Part print with two shaded views. Sizes in mm from the minimum x, y, z corner. A direction names the side the tool comes from. Coordinates: 2 decimals unless noted, no trailing zeros. Loops run counter-clockwise (first coordinate to the right, second up) from the corner with the lowest first, then second, coordinate; pieces in that order, holes last. Notation, with made-up numbers: (-3, 58) -> (11, 58) arc R26 cw to (11, 86) -> close; hole circle Ø3 at (-35, 83.25). An arc over 180 degrees is marked (long way). Write each question's results on one line, items separated by ' | '.
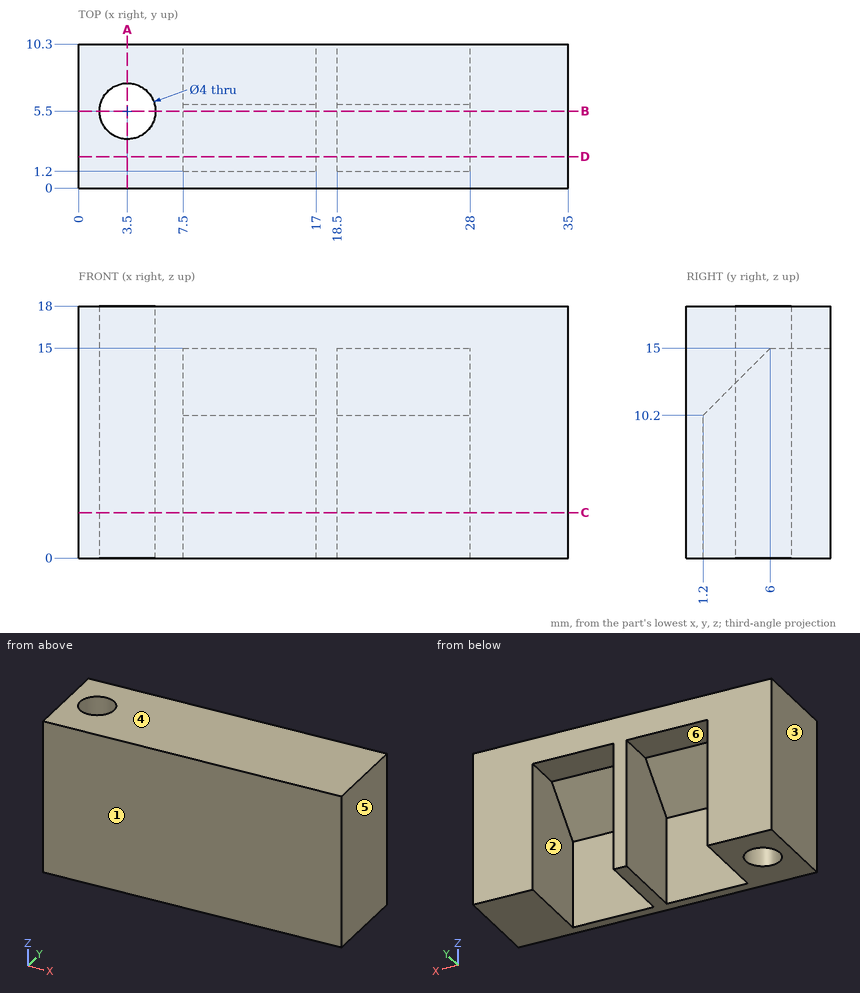
Q1. Drop flat-ended pins along their axis: pin 1 (5 mm diameter, centred on x = 12, z = 6, fed in from +Y); pin 2 (7.5 mm diameter, centred on x = 25, z = 4, fed in from +Y); pin 3 (2 mm diameter, centred on x = 13, y = 9, fed in from -Z); pin 4 (3 mm diameter, centred on x = 20.5, y = 4.5, fed in from -Z). Give the stop position or say it passes through.
Results are:
pin 1: y = 1.2 | pin 2: y = 10.3 | pin 3: z = 15 | pin 4: z = 12
Q2. Pull direction X, two halves, no side cores. Call the marked faces 3, 4, 5 and 6: +X half, -X half, draft (parallel to the pull), parting line (faces both ways), or undercut.
Results are:
face 3: -X half | face 4: draft | face 5: +X half | face 6: undercut
Q3. Cut at C-C on z = 3.25. Write the cut outline in (x, y).
Results are:
outline: (0, 0) -> (35, 0) -> (35, 10.3) -> (28, 10.3) -> (28, 1.2) -> (18.5, 1.2) -> (18.5, 10.3) -> (17, 10.3) -> (17, 1.2) -> (7.5, 1.2) -> (7.5, 10.3) -> (0, 10.3) -> close; hole circle Ø4 at (3.5, 5.5)
Q4. Cut at B-B on y = 5.5. Write the cut outline in (x, z).
Results are:
outline: (0, 0) -> (1.5, 0) -> (1.5, 18) -> (0, 18) -> close; (5.5, 0) -> (7.5, 0) -> (7.5, 14.5) -> (17, 14.5) -> (17, 0) -> (18.5, 0) -> (18.5, 14.5) -> (28, 14.5) -> (28, 0) -> (35, 0) -> (35, 18) -> (5.5, 18) -> close
Q5. Cut at D-D on y = 2.25. Write the cut outline in (x, z), and give its area (3 significant figures).
Results are:
outline: (0, 0) -> (7.5, 0) -> (7.5, 11.25) -> (17, 11.25) -> (17, 0) -> (18.5, 0) -> (18.5, 11.25) -> (28, 11.25) -> (28, 0) -> (35, 0) -> (35, 18) -> (0, 18) -> close | area: 416 mm^2
Q6. Cut at A-A on x = 3.5. Write the cut outline in (y, z).
Results are:
outline: (0, 0) -> (3.5, 0) -> (3.5, 18) -> (0, 18) -> close; (7.5, 0) -> (10.3, 0) -> (10.3, 18) -> (7.5, 18) -> close
Q7. Which spindle directions (+Z, -Z, +X, -X, +Y, -Y) get a long thin tool onto all of the face, cutting with end or side? Do the marked faces 1 and 2. Say none if no direction does.
Results are:
face 1: +Z, -Z, +X, -X, -Y | face 2: -Z, +Y
Q8. Wall check: L1, parallel to X at y = 5.5, z = 9.5; L2, parallel to X at y = 3, z = 10; L3, parallel to Y at x = 3.5, z = 14.25. Give the ranges that are in metal, low to high. Write a range as from..to.
Results are:
L1: 0..1.5, 5.5..7.5, 17..18.5, 28..35 | L2: 0..7.5, 17..18.5, 28..35 | L3: 0..3.5, 7.5..10.3
